Design review of the part built by this model. Coordinates are the model's own, in mm. Give positions to 0.01 mm unless a question says otherwise; leave off trailing zeros. Write each loop counter-clockwise with the first axis right and the second up, starting at its lowest first coordinate (ties: lowest second). Pieces come first, ordered by that corner, then holes. Notation, with made-up numbers: (44, 16) -> (79, 16) arc R20 cw to (79, 54) -> close; hole circle Ø1 at (44.5, 34). An arc over 180 degrees is marked (long way). Answer as a JSON object with one key per item and string values.
```python
from build123d import *

# Parameters (mm, degrees)
SKETCH1_R           = 1
BOSS_EXTRUDE1_DEPTH = 0.254
CUT_EXTRUDE1_DEPTH  = 1.254


with BuildPart() as part:
    # Sketch1 → Boss-Extrude1 (new body)
    with BuildSketch(Plane.XY):
        with BuildLine():
            Line((0, 4), (54.864, 4))
            ThreePointArc((54.864, 4), (58.864, 0), (54.864, -4))
            Line((54.864, -4), (0, -4))
            ThreePointArc((0, -4), (-4, 0), (0, 4))
        make_face()
        Circle(SKETCH1_R, mode=Mode.SUBTRACT)
        with Locations((54.864, 0)):
            Circle(SKETCH1_R, mode=Mode.SUBTRACT)
    extrude(amount=BOSS_EXTRUDE1_DEPTH)

    # Sketch2 → Cut-Extrude1 (cut, through all)
    with BuildSketch(Plane(origin=(0, 0, 0), x_dir=(-1, 0, 0), z_dir=(0, 0, -1))):
        with BuildLine():
            Line((-51.399898385, 2), (-3.464101615, 2))
            ThreePointArc((-3.464101615, 2), (-2, 3.464101615), (0, 4))
            Line((0, 4), (-54.864, 4))
            ThreePointArc((-54.864, 4), (-52.864, 3.464101615), (-51.399898385, 2))
        make_face()
        with BuildLine():
            Line((-51.399898385, -2), (-3.464101615, -2))
            ThreePointArc((-3.464101615, -2), (-2, -3.464101615), (0, -4))
            Line((0, -4), (-54.864, -4))
            ThreePointArc((-54.864, -4), (-52.864, -3.464101615), (-51.399898385, -2))
        make_face()
    extrude(amount=-CUT_EXTRUDE1_DEPTH, mode=Mode.SUBTRACT)


solid = part.part
```
(1) We need section B-B, the plane z = 0.1. State the section outline as (x, y) points, then the cut area to 3 significant figures.
Here are the results:
{"outline": "(3.46, -2) -> (51.4, -2) arc R4 ccw (long way) to (51.4, 2) -> (3.46, 2) arc R4 ccw (long way) to start; hole circle Ø2 at (0, 0); hole circle Ø2 at (54.86, 0)", "area": "283 mm²"}
(2) We need section C-C, the plane x = 17. State the section outline as (y, z) points, then the cut area to 3 significant figures.
Here are the results:
{"outline": "(-2, 0) -> (2, 0) -> (2, 0.25) -> (-2, 0.25) -> close", "area": "1.02 mm²"}
(3) We need section A-A, the plane y = 0. State the section outline as (x, z) points.
Here are the results:
{"outline": "(-4, 0) -> (-1, 0) -> (-1, 0.25) -> (-4, 0.25) -> close; (1, 0) -> (53.86, 0) -> (53.86, 0.25) -> (1, 0.25) -> close; (55.86, 0) -> (58.86, 0) -> (58.86, 0.25) -> (55.86, 0.25) -> close"}
(4) For line 1 along Y through (x, z) = (0, 0.2); line 2 along X through (y, z) = (0.25, 0.2); line 3 along X through (y, z) = (-2.75, 0.1), list the stretches that pass through material, from the lowest coordinate up.
Here are the results:
{"line 1": "y = -4 to -1, 1 to 4", "line 2": "x = -3.99 to -0.97, 0.97 to 53.9, 55.83 to 58.86", "line 3": "x = -2.9 to 2.9, 51.96 to 57.77"}
